Autodesk Inventor part; units mm, degrees
ref_plane "YZ Plane" through (0, 0, 0) normal (1, 0, 0) x (0, 1, 0)
ref_plane "XZ Plane" through (0, 0, 0) normal (0, 1, 0) x (-1, 0, 0)
ref_plane "XY Plane" through (0, 0, 0) normal (0, 0, 1) x (1, 0, 0)
sketch "Esboço1" plane through (0, 0, 0) normal (0, 0, 1) x (1, 0, 0)
  line L0 (5, -5) -> (-5, -5)
  line L1 (-5, -5) -> (-5, 5)
  line L2 (-5, 5) -> (-3.5, 5)
  line L3 (5, -3.5) -> (5, -5)
  line L4 (5, -5) -> (-5, 5) construction
  line L5 (-5, -5) -> (5, 5) construction
  line L6 (-3.5, 5) -> (-3.5, -3.5)
  line L7 (5, -3.5) -> (-3.5, -3.5)
  point P0 (0, 0)
  dimension "d0" = 10
  dimension "d1" = 10
  dimension "d2" = 1.5
  dimension "d4" = 5
  dimension "d5" = 5
extrude "Extrusão1" add sketch "Esboço1" along normal mid plane 10
fillet "Arredondamento1" radius 1 2 edges at (-3.5, 5, 0) (5, -3.5, 0)
hole "Furo1" at (1, -3.5, 0) direction (0, -1, 0) diameter 3 end through all
hole "Furo2" at (-3.5, 1, 0) direction (-1, 0, 0) diameter 3 end through all
properties part number "Cantoneira Gaveta" material "Liga de aço"
Could you check a few things on this model? Use its own coordinates, in mm. A direction names the side the tool comes from. Round coordinates to 2 decimals unless told otherwise and drop trailing zeros. Order: outer loops, then holes, each group sorted by start corner. A loop starts at its lowest first (then second) coordinate and runs counter-clockwise, first axis right, second up. Notation, with made-up numbers: M 61,76 L 108,76 A11 ccw 108,84 Z; hole C -25.5,13 d6. An arc over 180 degrees is marked long. One line per question, with ' | ' between items. Start each with the question number.
(1) Suppose I cut it at A-A on y = 1. List the corners of the cut face in (x, z) for me, then the cut area to 3 significant figures.
(2) For faces 1 (the face through (-3.5, -1, 0)), 2 (the face through (-4.26, 2.464, 0.325)), which set-ups out of +Z, -Z, +X, -X, +Y, -Y let a thin tool reach every point of the face, with its end or its side?
(3) Suppose I cut it at D-D on z = -1.75. List the corners of the cut face in (x, y) for me, then the cut area to 3 significant figures.
(4) For P1, Ø1, axis at x = -2.5, y = -1.5, coming from the +Z side; P2, Ø4, axis at y = 2, z = 2.5, coming from the +X side; P3, Ø2, axis at x = 2, z = -0.5, coming from the +Y side, each with a flat end and sliding along its axis, tell me the tip position at first contact or that it passes through.
(5) Suppose I cut it at C-C on z = 0. List the corners of the cut face in (x, y) for me.
(6) Thinking about a two-plate mould opening in Z: for faces 3 (the face through (-4, -2, -5)), 4 (the face through (-1, -5, 0)), 5 (the face through (2.464, -4.26, -0.325)), which applies, +Z half, -Z half, draft (parallel to the pull), parting line (faces both ways), or undercut?
(7) Please list where these lines run through material, in increasing order: line 1 along Z through (x, y) = (-3.9, 1); line 2 along X through (y, z) = (1.75, 4.25).
Geometry results:
1) outline: M -5,-5 L -3.5,-5 L -3.5,-1.5 L -5,-1.5 Z; M -5,1.5 L -3.5,1.5 L -3.5,5 L -5,5 Z | area: 10.5 mm²
2) face 1: +Z, -Z, +X, +Y | face 2: +X, -X
3) outline: M -5,-5 L 5,-5 L 5,-4.5 A1 ccw 4,-3.5 L -3.5,-3.5 L -3.5,4 A1 ccw -4.5,5 L -5,5 Z | area: 27.3 mm²
4) P1: through | P2: x = -3.5 | P3: y = -3.5
5) outline: M -5,-5 L -0.5,-5 L -0.5,-3.5 L -3.5,-3.5 L -3.5,-0.5 L -5,-0.5 Z; M -5,2.5 L -3.5,2.5 L -3.5,4 A1 ccw -4.5,5 L -5,5 Z; M 2.5,-5 L 5,-5 L 5,-4.5 A1 ccw 4,-3.5 L 2.5,-3.5 Z
6) face 3: -Z half | face 4: draft | face 5: undercut
7) line 1: -5 to -1.5, 1.5 to 5 | line 2: -5 to -3.5
